Geometry: final body of the model. Coordinates: model frame, mm. Face numbers are marked on the shaded views. Coordinates: 2 decimals unless noted, no trailing zeros. Write each loop counter-clockwise with the first axis right and the second up, starting at its lowest first coordinate (ties: lowest second). Pieces come first, ordered by that corner, then holes.
from build123d import *

# Parameters (mm, degrees)
BOX_W               = 20
BOX_H               = 15
BOX_DEPTH           = 10
SKETCH_R            = 2
POCKET_DEPTH        = 11
LINEARPATTERN_COUNT = 3
LINEARPATTERN_PITCH = 5


with BuildPart() as part:
    # Box → Box (new body)
    with BuildSketch(Plane.XY):
        with Locations((10, 7.5)):
            Rectangle(BOX_W, BOX_H)
    extrude(amount=BOX_DEPTH)

    # Sketch (on Face6 of BaseFeature) → Pocket (cut)
    with BuildSketch(Plane.XY.offset(10)):
        with Locations((5, 5)):
            Circle(SKETCH_R)
        with Locations((10, 5)):
            Circle(SKETCH_R)
        with Locations((15, 5)):
            Circle(SKETCH_R)
        with Locations((5, 11)):
            Circle(SKETCH_R)
        with Locations((10, 11)):
            Circle(SKETCH_R)
        with Locations((15, 11)):
            Circle(SKETCH_R)
    pocket = extrude(amount=-POCKET_DEPTH, mode=Mode.SUBTRACT)

    # LinearPattern: Pocket ×3
    with Locations(*[(i * LINEARPATTERN_PITCH, 0, 0) for i in range(1, LINEARPATTERN_COUNT)]):
        add(pocket, mode=Mode.SUBTRACT)


solid = part.part
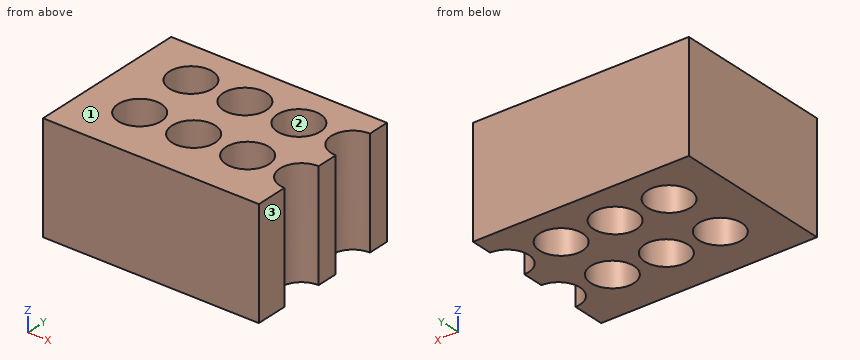
Item 1: Material intervals for probe 1 along Y at (x, z) = (15, 6); probe 2 along Y at (x, z) = (16.75, 9); probe 3 along X at (y, z) = (10.5, 7.75), sorted ascending.
Derived:
probe 1: y = 0 to 3, 7 to 9, 13 to 15
probe 2: y = 0 to 4.03, 5.97 to 10.03, 11.97 to 15
probe 3: x = 0 to 3.06, 6.94 to 8.06, 11.94 to 13.06, 16.94 to 18.06
Item 2: Pull-direction query (X, two-part tool) for the marked faces 1, 2 and 3; classes: released by +X, released by -X, zero draft, split by the parting line, or undercut.
Derived:
face 1: zero draft
face 2: undercut
face 3: released by +X
Item 3: Section C-C, the plane x = 10. Output: boundary loops of the cut face in (y, z).
Derived:
outline: (0, 0) - (3, 0) - (3, 10) - (0, 10) - close; (7, 0) - (9, 0) - (9, 10) - (7, 10) - close; (13, 0) - (15, 0) - (15, 10) - (13, 10) - close
Item 4: Pin query (flat end, axial travel): pin 1 (4 mm diameter, centred on y = 3.5, z = 3, fed in from +X); pin 2 (3 mm diameter, centred on x = 15, y = 11, fed in from -Z). Return the tip coordinate at first contact, or that it passes through.
Derived:
pin 1: stops at x = 20
pin 2: passes through
Item 5: Section A-A, the plane y = 11. Output: boundary loops of the cut face in (x, z), plus the area to 3 significant figures.
Derived:
outline: (0, 0) - (3, 0) - (3, 10) - (0, 10) - close; (7, 0) - (8, 0) - (8, 10) - (7, 10) - close; (12, 0) - (13, 0) - (13, 10) - (12, 10) - close; (17, 0) - (18, 0) - (18, 10) - (17, 10) - close
area: 60.0 mm2
Item 6: Section D-D, the plane x = 3.75. Output: boundary loops of the cut face in (y, z), plus the area to 4 significant figures.
Derived:
outline: (0, 0) - (3.44, 0) - (3.44, 10) - (0, 10) - close; (6.56, 0) - (9.44, 0) - (9.44, 10) - (6.56, 10) - close; (12.56, 0) - (15, 0) - (15, 10) - (12.56, 10) - close
area: 87.55 mm2
Item 7: Section B-B, the plane z = 6. Output: boundary loops of the cut face in (x, y).
Derived:
outline: (0, 0) - (20, 0) - (20, 3) arc R2 cw to (20, 7) - (20, 9) arc R2 cw to (20, 13) - (20, 15) - (0, 15) - close; hole circle Ø4 at (5, 5); hole circle Ø4 at (5, 11); hole circle Ø4 at (10, 5); hole circle Ø4 at (10, 11); hole circle Ø4 at (15, 5); hole circle Ø4 at (15, 11)
